```python
from build123d import *

# Parameters (mm, degrees)
SKETCH_1_R          = 15
EXTRUDE_1_DEPTH     = 3
SKETCH_2_R          = 8.5
EXTRUDE_2_DEPTH     = 20
SKETCH_3_R          = 10.332882869
SKETCH_3_R_2        = 7.5
CUT_EXTRUDE_1_DEPTH = 15
SKETCH_4_R          = 4
CUT_EXTRUDE_2_DEPTH = 37
CHAMFER_1_SIZE      = 2.8


with BuildPart() as part:
    # Эскиз1 → Бобышка-Вытянуть1 (new body)
    with BuildSketch(Plane.XY):
        Circle(SKETCH_1_R)
    extrude(amount=EXTRUDE_1_DEPTH)

    # Эскиз2 → Бобышка-Вытянуть2 (add)
    with BuildSketch(Plane.XY.offset(3)):
        Circle(SKETCH_2_R)
    extrude(amount=EXTRUDE_2_DEPTH)

    # Эскиз3 → Вырез-Вытянуть1 (cut)
    with BuildSketch(Plane.XY.offset(23)):
        Circle(SKETCH_3_R)
        Circle(SKETCH_3_R_2, mode=Mode.SUBTRACT)
    extrude(amount=-CUT_EXTRUDE_1_DEPTH, mode=Mode.SUBTRACT)

    # Эскиз4 → Вырез-Вытянуть2 (cut)
    with BuildSketch(Plane.XY.offset(23)):
        Circle(SKETCH_4_R)
    extrude(amount=-CUT_EXTRUDE_2_DEPTH, mode=Mode.SUBTRACT)

    # Фаска1
    chamfer_1_edges = [part.edges().sort_by_distance(p)[0] for p in [
        (-4, 0, 0),
    ]]
    chamfer(chamfer_1_edges, length=CHAMFER_1_SIZE)


solid = part.part
```
Source: CAD feature listing. Evaluate the final solid. Frame: model axes, mm. A direction names the side the tool comes from. Give positions to 0.01 mm unless a question says otherwise; leave off trailing zeros. Write each loop counter-clockwise with the first axis right and the second up, starting at its lowest first coordinate (ties: lowest second). Pieces come first, ordered by that corner, then holes. Notation, with made-up numbers: (35, 71) - (83, 71) arc R26 ccw to (83, 106) - close; hole circle Ø3 at (83.5, 19.5). An arc over 180 degrees is marked (long way). One line per item, written item: value. Start each with the question number.
Q1. Draft query along X for faces 3 (the face through (-7.493, 0.33, 15.605)), 4 (the face through (3.1, -6.5, 0)), 5 (the face through (3.821, -1.584, 2.664)). Return one class per face: +X half, -X half, draft (parallel to the pull), parting line (faces both ways), or undercut.
Q2. Material intervals for probe 1 along Y at (x, z) = (0, 14.75); probe 2 along Y at (x, z) = (0, 7); probe 3 along Z at (x, y) = (4.75, -6.5), sorted ascending. Write a range as from..to.
Q3. Section query D-D, the plane x = -8. Return the cut outline in (y, z).
Q4. Section query A-A, the plane x = 0. Return the cut outline in (y, z), then the cut area to 3 significant figures.
Q5. First-contact query: pin 1 Ø8 at (y, z) = (8.5, 17.5) entering from +X; pin 2 Ø8 at (y, z) = (-9.5, 16.5) entering from +X; pin 3 Ø12 at (y, z) = (2, 7.5) entering from +X; pin 4 Ø3 at (x, z) = (4.5, 6) entering from -Y. Flat tips, straight axial feed; report the tip coordinate or a pass-through.
Q6. Section query C-C, the plane z = 19. Return the cut outline in (x, y), then the cut area to 3 significant figures.
Q7. Set-up query: faces 1 (the face through (6.5, -6.5, 3)), 2 (the face through (-0.867, -3.905, 13.041)). Return all of +Z, -Z, +X, -X, +Y, -Y with unobstructed straight access to the full face (end or side cutting, diameter ignored); none if empty.
Answer:
1. face 3: parting line
1. face 4: draft
1. face 5: undercut
2. probe 1: y = -7.5..-4, 4..7.5
2. probe 2: y = -8.5..-4, 4..8.5
2. probe 3: z = 0..8
3. outline: (-12.69, 0) - (12.69, 0) - (12.69, 3) - (2.87, 3) - (2.87, 8) - (-2.87, 8) - (-2.87, 3) - (-12.69, 3) - close
4. outline: (-15, 0) - (-6.8, 0) - (-4, 2.8) - (-4, 23) - (-7.5, 23) - (-7.5, 8) - (-8.5, 8) - (-8.5, 3) - (-15, 3) - close; (4, 2.8) - (6.8, 0) - (15, 0) - (15, 3) - (8.5, 3) - (8.5, 8) - (7.5, 8) - (7.5, 23) - (4, 23) - close
4. area: 208 mm2
5. pin 1: stops at x = 6
5. pin 2: stops at x = 5.1
5. pin 3: stops at x = 15
5. pin 4: stops at y = -7.95
6. outline: circle Ø15 at (0, 0); hole circle Ø8 at (0, 0)
6. area: 126 mm2
7. face 1: +Z
7. face 2: +Z, -Z
